```python
from build123d import *

# Parameters (mm, degrees)
SKETCH1_W           = 508
SKETCH1_H           = 190.5
BOSS_EXTRUDE1_DEPTH = 6.35
SKETCH2_W           = 508
SKETCH2_H           = 190.5
SKETCH2_W_2         = 495.3
SKETCH2_H_2         = 177.8
BOSS_EXTRUDE2_DEPTH = 298.45
SKETCH3_W           = 6.35
SKETCH3_H           = 16.933333333
SKETCH3_H_2         = 16.933333334
CUT_EXTRUDE1_DEPTH  = 12.7
SKETCH4_W           = 6.35
SKETCH4_H           = 15.875
CUT_EXTRUDE2_DEPTH  = 6.35
SKETCH6_W           = 514.801062296
SKETCH6_H           = 254.881465808
CUT_EXTRUDE5_DEPTH  = 305.8
SKETCH5_W           = 6.35
SKETCH5_H           = 16.933333333
SKETCH5_H_2         = 16.933333334
CUT_EXTRUDE6_DEPTH  = 6.35
SKETCH7_W           = 6.35
SKETCH7_H           = 12.7
CUT_EXTRUDE7_DEPTH  = 7.35
SKETCH8_R           = 3.175
CUT_EXTRUDE8_DEPTH  = 7.35


with BuildPart() as part:
    # Sketch1 → Boss-Extrude1 (new body)
    with BuildSketch(Plane(origin=(0, 0, 0), x_dir=(1, 0, 0), z_dir=(0, 1, 0))):
        Rectangle(SKETCH1_W, SKETCH1_H)
    extrude(amount=BOSS_EXTRUDE1_DEPTH)

    # Sketch2 → Boss-Extrude2 (add)
    with BuildSketch(Plane(origin=(0, 6.35, 0), x_dir=(1, 0, 0), z_dir=(0, 1, 0))):
        Rectangle(SKETCH2_W, SKETCH2_H)
        Rectangle(SKETCH2_W_2, SKETCH2_H_2, mode=Mode.SUBTRACT)
    extrude(amount=BOSS_EXTRUDE2_DEPTH)

    # Sketch3 → Cut-Extrude1 (cut)
    with BuildSketch(Plane.XY.offset(95.25)):
        with BuildLine():
            Line((-3.302, 283.21), (-3.302, 6.35))
            Line((-3.302, 6.35), (3.302, 6.35))
            Line((3.302, 6.35), (3.302, 292.354))
            Line((3.302, 292.354), (-16.256, 292.354))
            Line((-16.256, 292.354), (-16.256, 285.75))
            Line((-16.256, 285.75), (-5.842, 285.75))
            ThreePointArc((-5.842, 285.75), (-4.045948776, 285.006051224), (-3.302, 283.21))
        make_face()
        with Locations((12.827, 80.433333334)):
            Rectangle(SKETCH3_W, SKETCH3_H)
        with Locations((12.827, 50.8)):
            Rectangle(SKETCH3_W, SKETCH3_H_2)
        with Locations((12.827, 21.166666667)):
            Rectangle(SKETCH3_W, SKETCH3_H)
    extrude(amount=-CUT_EXTRUDE1_DEPTH, mode=Mode.SUBTRACT)

    # Sketch4 → Cut-Extrude2 (cut)
    with BuildSketch(Plane.XY.offset(-88.9)):
        with Locations((-19.431, 284.1625)):
            Rectangle(SKETCH4_W, SKETCH4_H)
        with Locations((-19.431, 255.5875)):
            Rectangle(SKETCH4_W, SKETCH4_H)
        with Locations((-19.431, 227.0125)):
            Rectangle(SKETCH4_W, SKETCH4_H)
        with Locations((-19.431, 198.4375)):
            Rectangle(SKETCH4_W, SKETCH4_H)
        with Locations((-19.431, 169.8625)):
            Rectangle(SKETCH4_W, SKETCH4_H)
        with Locations((-19.431, 141.2875)):
            Rectangle(SKETCH4_W, SKETCH4_H)
        with Locations((-19.431, 112.7125)):
            Rectangle(SKETCH4_W, SKETCH4_H)
        with Locations((-19.431, 84.1375)):
            Rectangle(SKETCH4_W, SKETCH4_H)
        with Locations((-19.431, 55.5625)):
            Rectangle(SKETCH4_W, SKETCH4_H)
        with Locations((-19.431, 26.9875)):
            Rectangle(SKETCH4_W, SKETCH4_H)
    cut_extrude2 = extrude(amount=-CUT_EXTRUDE2_DEPTH, mode=Mode.SUBTRACT)

    # Mirror1: Cut-Extrude2 across plane
    add(cut_extrude2.mirror(Plane.ZY.offset(6.477)), mode=Mode.SUBTRACT)

    # Sketch6 → Cut-Extrude5 (cut, through all)
    with BuildSketch(Plane(origin=(0, 0, 0), x_dir=(1, 0, 0), z_dir=(0, 1, 0))):
        with Locations((9.750531148, -10.000845247)):
            Rectangle(SKETCH6_W, SKETCH6_H)
    extrude(amount=CUT_EXTRUDE5_DEPTH, mode=Mode.SUBTRACT)

    # Sketch5 → Cut-Extrude6 (cut)
    with BuildSketch(Plane(origin=(0, 0, 0), x_dir=(-1, 0, 0), z_dir=(0, -1, 0))):
        with Locations((250.825, -74.083333334)):
            Rectangle(SKETCH5_W, SKETCH5_H)
        with Locations((250.825, -44.45)):
            Rectangle(SKETCH5_W, SKETCH5_H_2)
        with Locations((250.825, -14.816666667)):
            Rectangle(SKETCH5_W, SKETCH5_H)
        with Locations((250.825, 14.816666667)):
            Rectangle(SKETCH5_W, SKETCH5_H)
        with Locations((250.825, 44.45)):
            Rectangle(SKETCH5_W, SKETCH5_H_2)
        with Locations((250.825, 74.083333334)):
            Rectangle(SKETCH5_W, SKETCH5_H)
    extrude(amount=-CUT_EXTRUDE6_DEPTH, mode=Mode.SUBTRACT)

    # Sketch7 → Cut-Extrude7 (cut, through all)
    with BuildSketch(Plane.ZY.offset(254)):
        with Locations((-92.075, 32.904545455)):
            Rectangle(SKETCH7_W, SKETCH7_H)
        with Locations((-92.075, 6.35)):
            Rectangle(SKETCH7_W, SKETCH7_H)
        with Locations((-92.075, 59.459090909)):
            Rectangle(SKETCH7_W, SKETCH7_H)
        with Locations((-92.075, 86.013636364)):
            Rectangle(SKETCH7_W, SKETCH7_H)
        with Locations((-92.075, 112.568181818)):
            Rectangle(SKETCH7_W, SKETCH7_H)
        with Locations((-92.075, 139.122727273)):
            Rectangle(SKETCH7_W, SKETCH7_H)
        with Locations((-92.075, 165.677272727)):
            Rectangle(SKETCH7_W, SKETCH7_H)
        with Locations((-92.075, 192.231818182)):
            Rectangle(SKETCH7_W, SKETCH7_H)
        with Locations((-92.075, 218.786363636)):
            Rectangle(SKETCH7_W, SKETCH7_H)
        with Locations((-92.075, 245.340909091)):
            Rectangle(SKETCH7_W, SKETCH7_H)
        with Locations((-92.075, 271.895454545)):
            Rectangle(SKETCH7_W, SKETCH7_H)
        with Locations((-92.075, 298.45)):
            Rectangle(SKETCH7_W, SKETCH7_H)
        with Locations((92.075, 298.45)):
            Rectangle(SKETCH7_W, SKETCH7_H)
        with Locations((92.075, 271.895454545)):
            Rectangle(SKETCH7_W, SKETCH7_H)
        with Locations((92.075, 245.340909091)):
            Rectangle(SKETCH7_W, SKETCH7_H)
        with Locations((92.075, 218.786363636)):
            Rectangle(SKETCH7_W, SKETCH7_H)
        with Locations((92.075, 192.231818182)):
            Rectangle(SKETCH7_W, SKETCH7_H)
        with Locations((92.075, 165.677272727)):
            Rectangle(SKETCH7_W, SKETCH7_H)
        with Locations((92.075, 139.122727273)):
            Rectangle(SKETCH7_W, SKETCH7_H)
        with Locations((92.075, 112.568181818)):
            Rectangle(SKETCH7_W, SKETCH7_H)
        with Locations((92.075, 86.013636364)):
            Rectangle(SKETCH7_W, SKETCH7_H)
        with Locations((92.075, 59.459090909)):
            Rectangle(SKETCH7_W, SKETCH7_H)
        with Locations((92.075, 32.904545455)):
            Rectangle(SKETCH7_W, SKETCH7_H)
        with Locations((92.075, 6.35)):
            Rectangle(SKETCH7_W, SKETCH7_H)
    extrude(amount=-CUT_EXTRUDE7_DEPTH, mode=Mode.SUBTRACT)

    # Sketch8 → Cut-Extrude8 (cut, through all)
    with BuildSketch(Plane.ZY.offset(254)):
        with Locations((0, 19.05)):
            Circle(SKETCH8_R)
    extrude(amount=-CUT_EXTRUDE8_DEPTH, mode=Mode.SUBTRACT)


solid = part.part
```
The model under review builds one solid part; all positions refer to its coordinate system, in mm. A direction names the side the tool comes from. Give positions to 0.01 mm unless a question says otherwise; leave off trailing zeros. Loops run counter-clockwise (first coordinate to the right, second up) from the corner with the lowest first, then second, coordinate; pieces in that order, holes last. Notation, with made-up numbers: (46, -10) - (88, -10) arc R34 cw to (88, 25) - close; hole circle Ø4 at (16, 61.25). An arc over 180 degrees is marked (long way). Answer as a JSON object with one key per item and string values.
Q1. Add section D-D on y = 193. State the section outline as (x, z) points, plus the area to 3 significant figures.
Worked out:
{"outline": "(-254, -88.9) - (-247.65, -88.9) - (-247.65, 88.9) - (-254, 88.9) - close", "area": "1,130 mm^2"}
Q2. Mouldability with a two-part tool opening along Z and no side actions: class faces 5 (the flat face through (-251, 3, -82.55)), 6 (the flat face through (-251, 33, 88.9)), 7 (the flat face through (-251, 245, -88.9)) as +Z half, -Z half, draft (parallel to the pull), parting line (faces both ways), or undercut.
Worked out:
{"face 5": "undercut", "face 6": "+Z half", "face 7": "-Z half"}
Q3. For faces 1 (the flat face through (-251, 212.436, 92)), 2 (the flat face through (-251, 86, -88.9)), 3 (the flat face through (-251, 292.1, 92)), 4 (the flat face through (-251, 6.35, 74)), list the 3-axis set-ups (+Z, -Z, +X, -X, +Y, -Y) from which the entire face can be reached by the end or side of a thin tool; tool diameter is ignored.
Worked out:
{"face 1": "+Z, +X, -X", "face 2": "-Z, +X, -X", "face 3": "+Z, +X, -X, +Y", "face 4": "+X, -X, -Y"}
Q4. Add section B-B on y = 19.05. State the section outline as (x, z) points (3 decimals), plus the area to 3 significant figures.
Worked out:
{"outline": "(-254, -95.25) - (-247.65, -95.25) - (-247.65, -3.175) - (-254, -3.175) - close; (-254, 3.175) - (-247.65, 3.175) - (-247.65, 95.25) - (-254, 95.25) - close", "area": "1,170 mm^2"}
Q5. Insertion check: pin 1 (1.9 mm diameter, centred on x = -252.5, z = 93, fed in from -Y); pin 2 (3 mm diameter, centred on x = -249, y = 298, fed in from -Z); pin 3 (2 mm diameter, centred on x = -249, z = 17, fed in from -Y). Each pin has a flat end and moves straight along its axis. Give the tip position at first contact, or say it passes through.
Worked out:
{"pin 1": "stops at y = 12.7", "pin 2": "stops at z = -88.9", "pin 3": "stops at y = 6.35"}
Q6. Add section A-A on z = 0. State the section outline as (x, y) points (3 decimals).
Worked out:
{"outline": "(-254, 0) - (-247.65, 0) - (-247.65, 15.875) - (-254, 15.875) - close; (-254, 22.225) - (-247.65, 22.225) - (-247.65, 304.8) - (-254, 304.8) - close"}
Q7. To check wall thickness, follow line 1 along Y through (x, z) = (-251.25, 0) (3 decimals); line 2 along Y through (x, z) = (-250.5, -41); line 3 along Z through (x, y) = (-250.5, 166). State the ranges of each line that lie inside material, in increasing order.
Worked out:
{"line 1": "y = 0 to 15.875, 22.225 to 304.8", "line 2": "y = 6.35 to 304.8", "line 3": "z = -88.9 to 88.9"}
Q8. Add section C-C on z = 68.5. State the section outline as (x, y) points, plus the area to 3 significant figures.
Worked out:
{"outline": "(-254, 6.35) - (-247.65, 6.35) - (-247.65, 304.8) - (-254, 304.8) - close", "area": "1,900 mm^2"}
